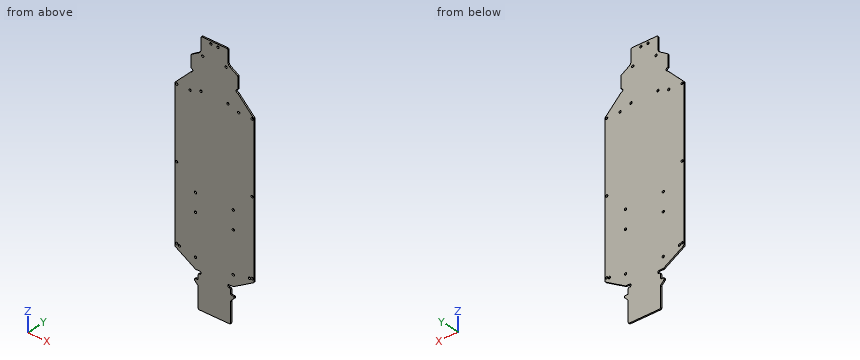
```python
from build123d import *

# Parameters (mm, degrees)
SKETCH2_R           = 1.25
BOSS_EXTRUDE1_DEPTH = 1.5


with BuildPart() as part:
    # Sketch2 → Boss-Extrude1 (new body)
    with BuildSketch(Plane(origin=(0, 0, 0), x_dir=(1, 0, 0), z_dir=(0, 1, 0))):
        with BuildLine():
            Line((44, -37.726695025), (44, -200.585786438))
            ThreePointArc((44, -200.585786438), (43.923879533, -200.96846987), (43.707106781, -201.292893219))
            Line((43.707106781, -201.292893219), (26, -219))
            ThreePointArc((26, -219), (24.105222952, -220.894777048), (26, -222.789554095))
            Line((26, -222.789554095), (26, -235.796673544))
            ThreePointArc((26, -235.796673544), (25.871071764, -236.287829305), (25.517532037, -236.652337374))
            Line((25.517532037, -236.652337374), (17.434936424, -241.540942021))
            ThreePointArc((17.434936424, -241.540942021), (15.667237789, -243.363482369), (15.022596611, -245.819261172))
            Line((15.022596611, -245.819261172), (15.022596611, -258))
            ThreePointArc((15.022596611, -258), (14.729703393, -258.707106781), (14.022596611, -259))
            Line((14.022596611, -259), (-13.977403389, -259))
            ThreePointArc((-13.977403389, -259), (-14.68451017, -258.707106781), (-14.977403389, -258))
            Line((-14.977403389, -258), (-14.977403389, -245.819261172))
            ThreePointArc((-14.977403389, -245.819261172), (-15.622044567, -243.363482369), (-17.389743201, -241.540942021))
            Line((-17.389743201, -241.540942021), (-25.472338815, -236.652337374))
            ThreePointArc((-25.472338815, -236.652337374), (-25.825878542, -236.287829305), (-25.954806777, -235.796673544))
            Line((-25.954806777, -235.796673544), (-25.954806777, -222.789554095))
            ThreePointArc((-25.954806777, -222.789554095), (-24.06002973, -220.894777048), (-25.954806777, -219))
            Line((-25.954806777, -219), (-43.661913558, -201.292893219))
            ThreePointArc((-43.661913558, -201.292893219), (-43.87868631, -200.96846987), (-43.954806777, -200.585786438))
            Line((-43.954806777, -200.585786438), (-43.954806777, -37.726695025))
            ThreePointArc((-43.954806777, -37.726695025), (-43.692021682, -36.735693323), (-42.972722404, -36.005112097))
            Line((-42.972722404, -36.005112097), (-21.448285322, -23.278417073))
            ThreePointArc((-21.448285322, -23.278417073), (-20.958022112, -23.070859537), (-20.430369695, -23))
            Line((-20.430369695, -23), (-15.977403389, -23))
            ThreePointArc((-15.977403389, -23), (-15.270296607, -22.707106781), (-14.977403389, -22))
            Line((-14.977403389, -22), (-14.977403389, -21))
            ThreePointArc((-14.977403389, -21), (-15.270296607, -20.292893219), (-15.977403389, -20))
            Line((-15.977403389, -20), (-16.977403389, -20))
            ThreePointArc((-16.977403389, -20), (-17.68451017, -19.707106781), (-17.977403389, -19))
            Line((-17.977403389, -19), (-17.977403389, -14.507024567))
            ThreePointArc((-17.977403389, -14.507024567), (-18.270296607, -13.799917786), (-18.977403389, -13.507024567))
            Line((-18.977403389, -13.507024567), (-21.477403389, -13.507024567))
            ThreePointArc((-21.477403389, -13.507024567), (-21.830956779, -13.360577958), (-21.977403389, -13.007024567))
            Line((-21.977403389, -13.007024567), (-21.977403389, -11.921238129))
            ThreePointArc((-21.977403389, -11.921238129), (-21.901282921, -11.538554697), (-21.68451017, -11.214131348))
            Line((-21.68451017, -11.214131348), (-18.563189826, -8.092811005))
            ThreePointArc((-18.563189826, -8.092811005), (-18.129644324, -7.443964307), (-17.977403389, -6.678597442))
            Line((-17.977403389, -6.678597442), (-17.977403389, 15))
            ThreePointArc((-17.977403389, 15), (-17.68451017, 15.707106781), (-16.977403389, 16))
            Line((-16.977403389, 16), (17.022596611, 16))
            ThreePointArc((17.022596611, 16), (17.729703393, 15.707106781), (18.022596611, 15))
            Line((18.022596611, 15), (18.022596611, -6.678597442))
            ThreePointArc((18.022596611, -6.678597442), (18.174837546, -7.443964307), (18.608383049, -8.092811005))
            Line((18.608383049, -8.092811005), (21.729703393, -11.214131348))
            ThreePointArc((21.729703393, -11.214131348), (21.946476144, -11.538554697), (22.022596611, -11.921238129))
            Line((22.022596611, -11.921238129), (22.022596611, -13.007024567))
            ThreePointArc((22.022596611, -13.007024567), (21.876150002, -13.360577958), (21.522596611, -13.507024567))
            Line((21.522596611, -13.507024567), (19.022596611, -13.507024567))
            ThreePointArc((19.022596611, -13.507024567), (18.31548983, -13.799917786), (18.022596611, -14.507024567))
            Line((18.022596611, -14.507024567), (18.022596611, -19))
            ThreePointArc((18.022596611, -19), (17.729703393, -19.707106781), (17.022596611, -20))
            Line((17.022596611, -20), (16.022596611, -20))
            ThreePointArc((16.022596611, -20), (15.31548983, -20.292893219), (15.022596611, -21))
            Line((15.022596611, -21), (15.022596611, -22))
            ThreePointArc((15.022596611, -22), (15.31548983, -22.707106781), (16.022596611, -23))
            Line((16.022596611, -23), (20.475562918, -23))
            ThreePointArc((20.475562918, -23), (21.003215334, -23.070859537), (21.493478545, -23.278417073))
            Line((21.493478545, -23.278417073), (43.017915627, -36.005112097))
            ThreePointArc((43.017915627, -36.005112097), (43.737214905, -36.735693323), (44, -37.726695025))
        make_face()
        with Locations(Location((42, -200, 0), (0, 0, 270))):
            Circle(SKETCH2_R, mode=Mode.SUBTRACT)
        with Locations(Location((27.091305327, -200, 0), (0, 0, 270))):
            Circle(SKETCH2_R, mode=Mode.SUBTRACT)
        with Locations(Location((4, -256, 0), (0, 0, 270))):
            Circle(SKETCH2_R, mode=Mode.SUBTRACT)
        with Locations(Location((13, -240, 0), (0, 0, 270))):
            Circle(SKETCH2_R, mode=Mode.SUBTRACT)
        with Locations(Location((15, -204, 0), (0, 0, 270))):
            Circle(SKETCH2_R, mode=Mode.SUBTRACT)
        with Locations(Location((42, -40, 0), (0, 0, 270))):
            Circle(SKETCH2_R, mode=Mode.SUBTRACT)
        with Locations(Location((39, -39, 0), (0, 0, 270))):
            Circle(SKETCH2_R, mode=Mode.SUBTRACT)
        with Locations(Location((21, -35, 0), (0, 0, 270))):
            Circle(SKETCH2_R, mode=Mode.SUBTRACT)
        with Locations(Location((42, -122, 0), (0, 0, 270))):
            Circle(SKETCH2_R, mode=Mode.SUBTRACT)
        with Locations(Location((21, -100, 0), (0, 0, 270))):
            Circle(SKETCH2_R, mode=Mode.SUBTRACT)
        with Locations(Location((21, -80, 0), (0, 0, 270))):
            Circle(SKETCH2_R, mode=Mode.SUBTRACT)
        with Locations(Location((-20.954806777, -80, 0), (0, 0, 270))):
            Circle(SKETCH2_R, mode=Mode.SUBTRACT)
        with Locations(Location((-20.954806777, -100, 0), (0, 0, 270))):
            Circle(SKETCH2_R, mode=Mode.SUBTRACT)
        with Locations(Location((-41.954806777, -122, 0), (0, 0, 270))):
            Circle(SKETCH2_R, mode=Mode.SUBTRACT)
        with Locations(Location((-20.954806777, -35, 0), (0, 0, 270))):
            Circle(SKETCH2_R, mode=Mode.SUBTRACT)
        with Locations(Location((-38.954806777, -39, 0), (0, 0, 270))):
            Circle(SKETCH2_R, mode=Mode.SUBTRACT)
        with Locations(Location((-41.954806777, -40, 0), (0, 0, 270))):
            Circle(SKETCH2_R, mode=Mode.SUBTRACT)
        with Locations(Location((-14.954806777, -204, 0), (0, 0, 270))):
            Circle(SKETCH2_R, mode=Mode.SUBTRACT)
        with Locations(Location((-12.954806777, -240, 0), (0, 0, 270))):
            Circle(SKETCH2_R, mode=Mode.SUBTRACT)
        with Locations(Location((-3.954806777, -256, 0), (0, 0, 270))):
            Circle(SKETCH2_R, mode=Mode.SUBTRACT)
        with Locations(Location((-27.046112104, -200, 0), (0, 0, 270))):
            Circle(SKETCH2_R, mode=Mode.SUBTRACT)
        with Locations(Location((-41.954806777, -200, 0), (0, 0, 270))):
            Circle(SKETCH2_R, mode=Mode.SUBTRACT)
    extrude(amount=BOSS_EXTRUDE1_DEPTH)


solid = part.part
```
Input: part model. Units: mm. Frame: model coordinates. Give positions to 0.01 mm unless a question says otherwise; leave off trailing zeros. Put each result on its own line as item: value.
Item 1: Section query A-A, the plane y = 0.95. Count the separate pieces of the cut face and the enclosed holes in it, then the cut area to 3 significant figures.
Found:
separate pieces: 1
enclosed holes: 22
area: 19,600 mm^2
Item 2: Contact query for flat-ended pins moving along their axis: pin 1 (0.8 mm diameter, centred on y = 1, z = 226.5, fed in from +X); pin 2 (0.5 mm diameter, centred on y = 1, z = 12.5, fed in from +X). Output: stop coordinate, or through.
Found:
pin 1: stops at x = 26
pin 2: stops at x = 22.02
Item 3: Ray query, L1, parallel to X at y = 0.6, z = 100; L2, parallel to Z at x = -21.5, y = 1.4; L3, parallel to X at y = 1.25, z = 122. Return the intervals inside material, ascending. Write a range as from..to.
Found:
L1: x = -43.95..-22.2, -19.7..19.75, 22.25..44
L2: z = 11.03..13.51, 23.31..33.88, 36.12..78.88, 81.12..98.88, 101.12..239.05
L3: x = -43.95..-43.2, -40.7..40.75, 43.25..44
